Answer from the drawing. Dimensions are ordinates in mm from the lowest x, y and z of the part. A direction names the side the tool comes from. Give positions to 0.01 mm unless a question says otherwise; leave off trailing zeros. Order: outer loops, then holes, each group sorted by start corner. A loop starts at its lowest first (then second) coordinate and runs counter-clockwise, first axis right, second up.
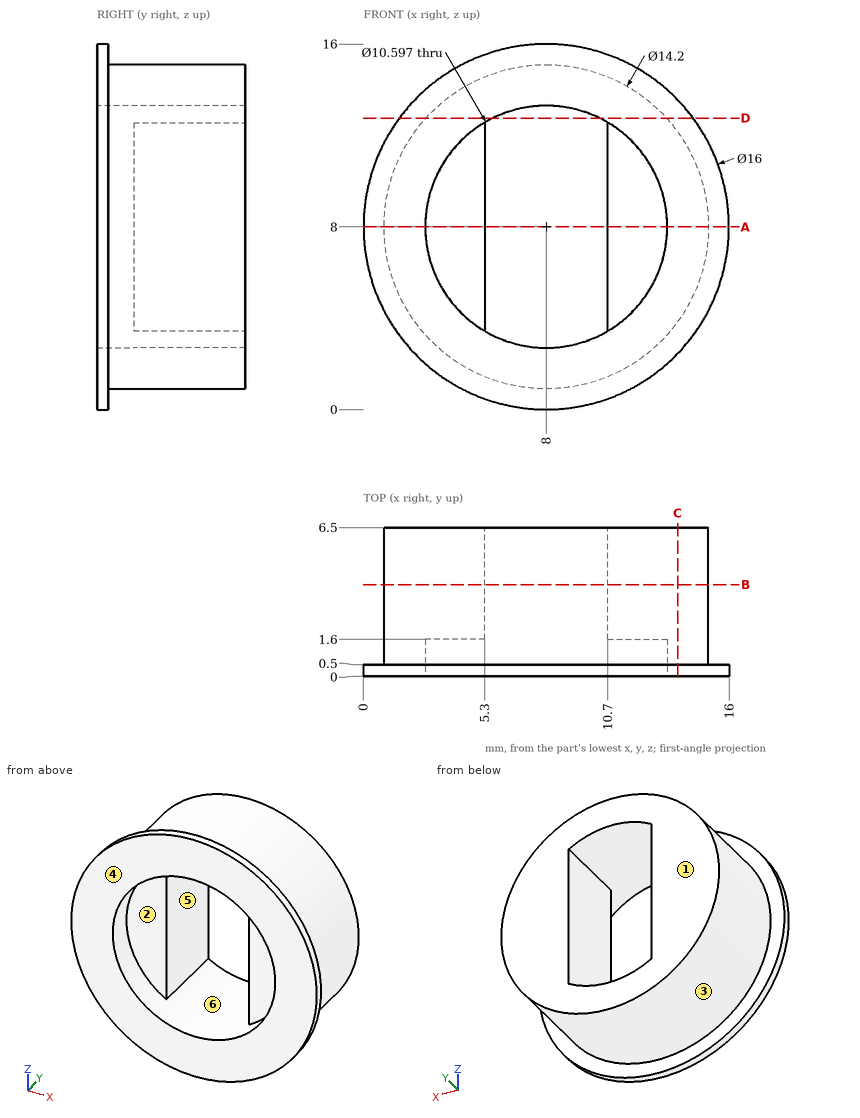
1. The mould has two halves that part along Z. Classify the marked faces 1, 2 and 3: pulls with the +Z half, pulls with the -Z half, needs draft (parallel to the pull), parting line crosses it, or undercut.
Findings below:
face 1: needs draft
face 2: undercut
face 3: parting line crosses it
2. Which of the six approach directions +Z, -Z, +X, -X, +Y, -Y give full straight-line access (tool end or side, diameter ignored) to the marked faces 4, 5 and 6?
Findings below:
face 4: +Z, -Z, +X, -X, -Y
face 5: +Y, -Y
face 6: -Y
3. The part is cut by section B-B (y = 4). Write down the section's boundary in (x, z).
Findings below:
outline: circle Ø14.2 at (8, 8); hole (5.3, 3.44) arc R5.3 ccw to (10.7, 3.44) - (10.7, 12.56) arc R5.3 ccw to (5.3, 12.56) - close
4. The part is cut by section C-C (x = 13.75). Write down the section's boundary in (y, z) (1 decimal).
Findings below:
outline: (0, 2.4) - (0.5, 2.4) - (0.5, 3.8) - (6.5, 3.8) - (6.5, 12.2) - (0.5, 12.2) - (0.5, 13.6) - (0, 13.6) - close
5. Given P1, Ø0.8, axis at x = 12, z = 9, coming from the -Y side, flat-ended and moving along its own axis, determine where the tip first touches the part or whether it passes through.
Findings below:
P1: stops at y = 1.6
6. The part is cut by section D-D (z = 12.75). Write down the section's boundary in (x, y).
Findings below:
outline: (1.56, 0) - (5.65, 0) - (5.65, 6.5) - (2.72, 6.5) - (2.72, 0.5) - (1.56, 0.5) - close; (10.35, 0) - (14.44, 0) - (14.44, 0.5) - (13.28, 0.5) - (13.28, 6.5) - (10.35, 6.5) - close
7. The part is cut by section A-A (z = 8). Write down the section's boundary in (x, y).
Findings below:
outline: (0, 0) - (2.7, 0) - (2.7, 1.6) - (5.3, 1.6) - (5.3, 6.5) - (0.9, 6.5) - (0.9, 0.5) - (0, 0.5) - close; (10.7, 1.6) - (13.3, 1.6) - (13.3, 0) - (16, 0) - (16, 0.5) - (15.1, 0.5) - (15.1, 6.5) - (10.7, 6.5) - close
8. Straight lines are drawn through the part: probe 1 along X at (y, z) = (1.5, 8); probe 2 along X at (y, z) = (3, 8); probe 3 along Y at (x, z) = (4.25, 9). For each, find the intervals that lie inside material, in ascending order.
Findings below:
probe 1: x = 0.9 to 2.7, 13.3 to 15.1
probe 2: x = 0.9 to 5.3, 10.7 to 15.1
probe 3: y = 1.6 to 6.5
